Can you work these out from the model? Positions are in its coordinate system, mm. A direction names the side the tool comes from. Coordinates: 2 decimals unless noted, no trailing zeros. Order: outer loops, then holes, each group sorted by start corner. A loop starts at its lowest first (then second) coordinate and runs counter-clockwise, first axis right, second up. Notation, with made-up numbers: (-9.5, 73.5) -> (10.5, 73.5) arc R17 cw to (10.5, 101.5) -> close; hole circle Ø11 at (3, 46). An arc over 180 degrees is marked (long way). Answer as CSV lines item,"result".
from build123d import *

# Parameters (mm, degrees)
F1_DEPTH = 3.175
F0_W     = 482.6
F0_H     = 3.175
F2_DEPTH = 38.1


with BuildPart() as f1:
    # F0 (on Top) → F1 (new body)
    with BuildSketch(Plane.XY):
        with BuildLine():
            Line((-241.3, -23.8125), (241.3, -23.8125))
            Line((241.3, -23.8125), (241.3, 23.8125))
            Line((241.3, 23.8125), (212.6702423383, 23.8125))
            ThreePointArc((212.6702423383, 23.8125), (120.65, -20.6375), (28.6297576617, 23.8125))
            Line((28.6297576617, 23.8125), (-28.6297576617, 23.8125))
            ThreePointArc((-28.6297576617, 23.8125), (-120.65, -20.6375), (-212.6702423383, 23.8125))
            Line((-212.6702423383, 23.8125), (-241.3, 23.8125))
            Line((-241.3, 23.8125), (-241.3, -23.8125))
        make_face()
    extrude(amount=-F1_DEPTH)

    # F0 (on Top) → F2 (join)
    with BuildSketch(Plane.XY):
        with Locations((0, -25.4)):
            Rectangle(F0_W, F0_H)
    extrude(amount=-F2_DEPTH)


solid = f1.part
Q1. If I drill on line 1 (X direction, y = 4, z = -1.5); line 2 (Y direction, x = -159, z = -19); line 3 (Z direction, x = -219.5, y = 14) (3 decimals), over which ranges is the centre line in solid material (lowest first)?
Solution:
line 1,"-241.3 to -192.63, -48.67 to 48.67, 192.63 to 241.3"
line 2,"-26.99 to -23.81"
line 3,"-3.175 to 0"
Q2. Imagine slicing it at A-A (y = 13). List the corners of the cut face in (x, z) for me (3 decimals).
Solution:
outline,"(-241.3, -3.175) -> (-202.94, -3.175) -> (-202.94, 0) -> (-241.3, 0) -> close; (-38.36, -3.175) -> (38.36, -3.175) -> (38.36, 0) -> (-38.36, 0) -> close; (202.94, -3.175) -> (241.3, -3.175) -> (241.3, 0) -> (202.94, 0) -> close"
Q3. We'd pull the mould along X, two halves only. Please class faces 3 (the flat face through (241.3, -13, -2)), 4 (the flat face through (-3, -5, -3.175)), 5 (the cylindrical face through (-119.17, -20.63, -1.57)): pulls with the +X half, pulls with the -X half, needs draft (parallel to the pull), parting line crosses it, or undercut.
Solution:
face 3,"pulls with the +X half"
face 4,"needs draft"
face 5,"undercut"
Q4. Imagine slicing it at C-C (z = -19). List the corners of the cut face in (x, y) for me.
Solution:
outline,"(-241.3, -26.99) -> (241.3, -26.99) -> (241.3, -23.81) -> (-241.3, -23.81) -> close"
Q5. Which directions (+Z, -Z, +X, -X, +Y, -Y) give clear straight access to the entire face, cutting with the end or side of a thin tool? Please do faces 1 (the flat face through (-3, -23.812, -20)), 2 (the flat face through (-3, -7, 0)).
Solution:
face 1,"-Z, +X, -X, +Y"
face 2,"+Z, +X, -X, +Y, -Y"
Q6. For P1, Ø24, axis at x = 98, y = -11.5, coming from the -Z side (3 decimals); P2, Ø4, axis at x = -81, z = -13.5, coming from the +Y side, each with a flat end and sliding along its axis, tell me the tip position at first contact or that it passes through.
Solution:
P1,"z = -3.175"
P2,"y = -23.81"
Q7. Imagine slicing it at D-D (y = -13). List the corners of the cut face in (x, z) for me (3 decimals), and give its area (3 significant figures).
Solution:
outline,"(-241.3, -3.175) -> (-162.317, -3.175) -> (-162.317, 0) -> (-241.3, 0) -> close; (-78.983, -3.175) -> (78.983, -3.175) -> (78.983, 0) -> (-78.983, 0) -> close; (162.317, -3.175) -> (241.3, -3.175) -> (241.3, 0) -> (162.317, 0) -> close"
area,"1,000 mm2"
Q8. Imagine slicing it at B-B (x = -163). List the corners of the cut face in (y, z) for me (1 decimal).
Solution:
outline,"(-27, -38.1) -> (-23.8, -38.1) -> (-23.8, -3.2) -> (-12.7, -3.2) -> (-12.7, 0) -> (-27, 0) -> close"
